from build123d import *

# Parameters (mm, degrees)
F1_DEPTH = 47.625
F3_DEPTH = 6.35
F4_R     = 0.508


# Not quite as in the source:
# - a pattern or mirror of a feature is missing from the dataset's text; its kind, count and spacing are read off the source's solid


with BuildPart() as f1:
    # F0 (on Front) → F1 (new body, symmetric)
    with BuildSketch(Plane.XZ):
        Polygon((20.8971929933, 0), (41.7943859866, 36.195), (35.9285072517, 36.195), (17.9642536258, 5.08), (-17.9642536258, 5.08), (-35.9285072517, 36.195), (-41.7943859866, 36.195), (-20.8971929933, 0), align=None)
    extrude(amount=F1_DEPTH, both=True)

    # F2 (on Right) → F3 (join, symmetric)
    with BuildSketch(Plane.YZ):
        Polygon((-47.625, 1.524), (-51.308, 1.524), (-51.308, 2.286), (-52.07, 2.286), (-54.0561154682, 0.762), (-54.0561154682, 0), (-47.625, 0), align=None)
    f3 = extrude(amount=F3_DEPTH, both=True)

    # F3_copies: F3 across plane
    add(f3.mirror(Plane.ZX))

    # F4
    f4_edges = [f1.edges().sort_by_distance(p)[0] for p in [
        (-6.35, -47.625, 0.762),
        (6.35, -47.625, 0.762),
        (0, -47.625, 1.524),
        (6.35, 47.625, 0.762),
        (0, 47.625, 1.524),
        (-6.35, 47.625, 0.762),
    ]]
    fillet(f4_edges, radius=F4_R)


solid = f1.part
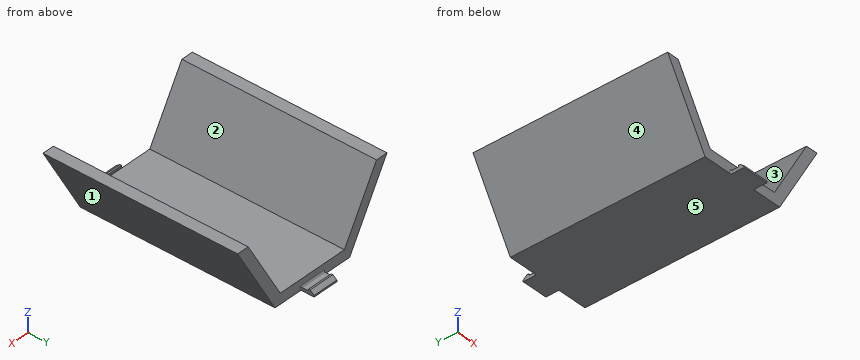
Here's how the part is built. I have some questions about the finished solid (model axes, mm). Face numbers are marked on the shaded views. A direction names the side the tool comes from. Give positions to 0.01 mm unless a question says otherwise; leave off trailing zeros. Loops run counter-clockwise (first coordinate to the right, second up) from the corner with the lowest first, then second, coordinate; pieces in that order, holes last. Notation, with made-up numbers: (-11, -9.5) -> (-1, -9.5) arc R20 ccw to (-1, 5.5) -> close; hole circle Ø5 at (-38, 71.25). An arc over 180 degrees is marked (long way). Answer as a JSON object with one key per item and string values. Group by question number.
Item 1: Will these pins go through, and if not, where does the flat tip stop? pin 1 (2.5 mm diameter, centred on y = 51, z = 1, fed in from +X); pin 2 (5 mm diameter, centred on x = 7.5, y = -13, fed in from +Z); pin 3 (8 mm diameter, centred on y = 21.5, z = 32, fed in from -X); pin 4 (11 mm diameter, centred on x = 0.5, z = 13.5, fed in from -Y).
Item 2: Imagine slicing it at D-D on x = 25. Write out the boundary of the cut face in (y, z) (3 decimals), then the cut area to 3 significant figures.
Item 3: Thinking about a two-plate mould opening in X: for the marked faces 3, 4 and 5, which applies, pulls with the +X half, pulls with the -X half, needs draft (parallel to the pull), parting line crosses it, or undercut?
Item 4: Imagine slicing it at B-B on z = 9. Write out the boundary of the cut face in (x, y) (3 decimals), then the cut area to 3 significant figures.
Item 5: I need wall thicknesses on L1, parallel to Z at x = -19, y = 31; L2, parallel to Z at x = 0, y = 23; L3, parallel to X at y = -31, z = 17. Which ranges of each line are inside material? Lowest first, please.
Item 6: Imagine slicing it at A-A on y = 39.5. Write out the boundary of the cut face in (x, z) (1 decimal).
Item 7: Imagine slicing it at C-C on x = -15. Write out the boundary of the cut face in (y, z) (3 decimals), then the cut area to 3 significant figures.
Item 8: On a 3-axis mill with a long thin cutter (end or side, diameter ignored), from which of +Z, -Z, +X, -X, +Y, -Y can I reach the whole of each face in a straight line? I mean the marked faces 1 and 2. Say none if no direction works.
Answer list:
{
 "1": {"pin 1": "stops at x = 6.35", "pin 2": "stops at z = 5.08", "pin 3": "stops at x = -41.68", "pin 4": "passes through"},
 "2": {"outline": "(-47.625, 7.106) -> (47.625, 7.106) -> (47.625, 17.266) -> (-47.625, 17.266) -> close", "area": "968 mm2"},
 "3": {"face 3": "undercut", "face 4": "pulls with the -X half", "face 5": "needs draft"},
 "4": {"outline": "(-26.093, -47.625) -> (-20.227, -47.625) -> (-20.227, 47.625) -> (-26.093, 47.625) -> close; (20.227, -47.625) -> (26.093, -47.625) -> (26.093, 47.625) -> (20.227, 47.625) -> close", "area": "1,120 mm2"},
 "5": {"L1": "z = 0 to 6.87", "L2": "z = 0 to 5.08", "L3": "x = -30.71 to -24.85, 24.85 to 30.71"},
 "6": {"outline": "(-41.8, 36.2) -> (-20.9, 0) -> (20.9, 0) -> (41.8, 36.2) -> (35.9, 36.2) -> (18, 5.1) -> (-18, 5.1) -> (-35.9, 36.2) -> close"},
 "7": {"outline": "(-47.625, 0) -> (47.625, 0) -> (47.625, 5.08) -> (-47.625, 5.08) -> close", "area": "484 mm2"},
 "8": {"face 1": "-Z, +X, +Y, -Y", "face 2": "+Z, +Y, -Y"}
}
